Verification items for the finished model (mm, model axes). A direction names the side the tool comes from. Coordinates: 2 decimals unless noted, no trailing zeros. Order: outer loops, then holes, each group sorted by start corner. A loop starts at its lowest first (then second) coordinate and runs counter-clockwise, first axis right, second up. Notation, with made-up numbers: M -31.5,46 L -17.5,46 A13 cw -17.5,59 Z; hole C -30.75,34.25 d8. An arc over 180 degrees is marked long. Answer as a JSON object with one key per item and string values. Group by question number.
(1) Cross-section at B-B (x = 0). Count the separate pieces of the cut face and the enclosed holes in it, plus the area to 3 significant figures.
(2) Gauge pin test, flat ends, axial feed: pin 1 Ø2 at (x, y) = (10, 19) entering from -Z; pin 2 Ø4 at (x, y) = (-8.5, 31.5) entering from +Z; pin 3 Ø1.5 at (x, z) = (0.5, -0.5) entering from -Y; pin 4 Ø4.5 at (x, z) = (-0.5, -1) entering from +Y. Record the tip position at first contact, or that the pin passes through.
(3) Cross-section at C-C (y = 26). Enter the section's corners in (x, z), plus the area to 3 significant figures.
(4) Mould release check, pull along Y, two halves, no side actions. Record for faces 1 (the face through (9.911, 40.014, -4.015)), 2 (the face through (5, 21, 0)), 3 (the face through (-2, 33.5, 4)): released by +Y, released by -Y, zero draft, split by the parting line, or undercut.
(5) Cross-section at A-A (y = 38.5). Enter the section's corners in (x, z) (3 decimals).
(6) Material ranges on line 1 (Z direction, x = 0, y = 40.2) (3 decimals); line 2 (Y direction, x = -2.25, z = 5.5); line 3 (X direction, y = 19.75, z = 0), recorded low to high.
(7) Access from +Z, -Z, +X, -X, +Y, -Y to the whole of each face (thin tool, end or side, straight path). Record for faces 4 (the face through (-11.99, 6.49, 0.53)), 5 (the face through (5, 18, 0)), 6 (the face through (-9.48, 40.01, -6.44)).
from build123d import *

# Parameters (mm, degrees)
CROQUIS3_R              = 12
CROQUIS3_R_2            = 3.25
SALIENTE_EXTRUIR1_DEPTH = 1
MATRIZL1_COUNT          = 8
MATRIZL1_PITCH          = 3
CROQUIS5_R              = 1.55
CORTAR_EXTRUIR1_DEPTH   = 2
MATRIZC1_COUNT          = 6
CHAFL_N3_SIZE           = 0.3
CHAFL_N3_SIZE2          = 0.519615242
CROQUIS6_R              = 7.15
CORTAR_EXTRUIR2_DEPTH   = 1
CHAFL_N2_SIZE           = 0.15
CHAFL_N2_SIZE2          = 0.259807621
CHAFL_N4_SIZE           = 1
CHAFL_N4_SIZE2          = 1.732050808


with BuildPart() as part:
    # Croquis1 → Revolución1 (revolve)
    with BuildSketch(Plane.XY):
        Polygon((0, 0), (6, 0), (6, 9), (5.25, 9), (5.25, 12), (4.75, 12), (4.75, 22), (8, 22), (8, 39), (12.5, 39), (12.5, 41), (0, 41), align=None)
    revolve(axis=Axis((0, 41, 0), (0, -1, 0)))

    # Croquis2 → Cortar-Revolución1 (revolve, cut)
    with BuildSketch(Plane.XY):
        Polygon((0, 0), (2.5, 0), (2.5, 12), (1.7, 12), (1.7, 14), (3.25, 14), (3.25, 33.5), (5.25, 33.5), (5.25, 36), (6.725, 36), (6.725, 41), (0, 41), align=None)
    revolve(axis=Axis((0, 0, 0), (0, 1, 0)), mode=Mode.SUBTRACT)

    # Croquis3 → Saliente-Extruir1 (add)
    with BuildSketch(Plane.XZ):
        Circle(CROQUIS3_R)
        Circle(CROQUIS3_R_2, mode=Mode.SUBTRACT)
    saliente_extruir1 = extrude(amount=-SALIENTE_EXTRUIR1_DEPTH)

    # MatrizL1: Saliente-Extruir1 ×8
    with Locations(*[(0, i * MATRIZL1_PITCH, 0) for i in range(1, MATRIZL1_COUNT)]):
        add(saliente_extruir1)

    # Croquis5 → Cortar-Extruir1 (cut)
    with BuildSketch(Plane(origin=(0, 41, 0), x_dir=(1, 0, 0), z_dir=(0, 1, 0))):
        with Locations((0, 10.125)):
            Circle(CROQUIS5_R)
    cortar_extruir1 = extrude(amount=-CORTAR_EXTRUIR1_DEPTH, mode=Mode.SUBTRACT)

    # MatrizC1: Cortar-Extruir1 ×6 about axis
    matrizc1_axis = Axis((0, 0, 0), (0, 1, 0))
    for i in range(1, MATRIZC1_COUNT):
        add(cortar_extruir1.rotate(matrizc1_axis, i * 360 / MATRIZC1_COUNT), mode=Mode.SUBTRACT)

    # Chaflán3
    chafl_n3_edges = [part.edges().sort_by_distance(p)[0] for p in [
        (-1.7, 14, 0),
    ]]
    chafl_n3_side = [part.faces().sort_by_distance(p)[0] for p in [
        (-1.791923882, 14, 0),
    ]]
    chamfer(chafl_n3_edges, length=CHAFL_N3_SIZE, length2=CHAFL_N3_SIZE2, reference=chafl_n3_side[0])

    # Croquis6 → Cortar-Extruir2 (cut)
    with BuildSketch(Plane(origin=(0, 41, 0), x_dir=(1, 0, 0), z_dir=(0, 1, 0))):
        Circle(CROQUIS6_R)
    extrude(amount=-CORTAR_EXTRUIR2_DEPTH, mode=Mode.SUBTRACT)

    # Chaflán2
    chafl_n2_edges = [part.edges().sort_by_distance(p)[0] for p in [
        (-1.7, 12, 0),
    ]]
    chafl_n2_side = [part.faces().sort_by_distance(p)[0] for p in [
        (-2.429289322, 12, 0),
    ]]
    chamfer(chafl_n2_edges, length=CHAFL_N2_SIZE, length2=CHAFL_N2_SIZE2, reference=chafl_n2_side[0])

    # Chaflán4
    chafl_n4_edges = [part.edges().sort_by_distance(p)[0] for p in [
        (-3.25, 33.5, 0),
    ]]
    chafl_n4_side = [part.faces().sort_by_distance(p)[0] for p in [
        (-3.398492424, 33.5, 0),
    ]]
    chamfer(chafl_n4_edges, length=CHAFL_N4_SIZE, length2=CHAFL_N4_SIZE2, reference=chafl_n4_side[0])


solid = part.part
Taken from the geometry:
{
 "1": {"separate pieces": "4", "enclosed holes": "0", "area": "362 mm²"},
 "2": {"pin 1": "stops at z = -7.94", "pin 2": "stops at z = 4.66", "pin 3": "passes through", "pin 4": "stops at y = 31.97"},
 "3": {"outline": "C 0,0 d16; hole C 0,0 d6.5", "area": "168 mm²"},
 "4": {"face 1": "zero draft", "face 2": "undercut", "face 3": "released by +Y"},
 "5": {"outline": "C 0,0 d16; hole C 0,0 d13.45"},
 "6": {"line 1": "z = -12.5 to -11.675, -8.575 to -7.15, 7.15 to 8.575, 11.675 to 12.5", "line 2": "y = 0 to 10, 12 to 13, 15 to 16, 18 to 19, 21 to 36", "line 3": "x = -4.75 to -3.25, 3.25 to 4.75"},
 "7": {"face 4": "-Y", "face 5": "none", "face 6": "+Y"}
}
